```python
from build123d import *

# Parameters (mm, degrees)
SKETCH1_W           = 55.88
SKETCH1_H           = 9.981767046
SKETCH1_R           = 2.0193
BOSS_EXTRUDE1_DEPTH = 2.54
SKETCH2_W           = 55.88
SKETCH2_H           = 1.152145831
BOSS_EXTRUDE2_DEPTH = 17.78
SKETCH3_W           = 1.2265406
SKETCH3_H           = 17.78
SKETCH3_W_2         = 1.1438128
BOSS_EXTRUDE4_DEPTH = 6.35
SKETCH4_R           = 1.524
CUT_EXTRUDE1_DEPTH  = 105.035332272
CUT_EXTRUDE3_DEPTH  = 105.035332272
BOSS_EXTRUDE5_DEPTH = 2.54
BOSS_EXTRUDE6_DEPTH = 2.54
FILLET1_R           = 2.3368
FILLET2_R           = 2.3368
FILLET3_R           = 2.3368
FILLET4_R           = 2.3368
BOSS_EXTRUDE7_START = 2.54
SKETCH8_R           = 1.524
BOSS_EXTRUDE7_DEPTH = 2.54


with BuildPart() as part:
    # Sketch1 → Boss-Extrude1 (new body)
    with BuildSketch(Plane.XY):
        with Locations((-73.708835459, 211.206122276)):
            Rectangle(SKETCH1_W, SKETCH1_H)
        with Locations((-96.565388679, 211.879005799)):
            Circle(SKETCH1_R, mode=Mode.SUBTRACT)
        with Locations((-50.848835459, 211.879005799)):
            Circle(SKETCH1_R, mode=Mode.SUBTRACT)
    extrude(amount=BOSS_EXTRUDE1_DEPTH)

    # Sketch2 → Boss-Extrude2 (add)
    with BuildSketch(Plane.XY.offset(2.54)):
        with Locations((-73.708835459, 206.791311669)):
            Rectangle(SKETCH2_W, SKETCH2_H)
    extrude(amount=BOSS_EXTRUDE2_DEPTH)

    # Sketch3 → Boss-Extrude4 (add)
    with BuildSketch(Plane(origin=(0, 207.367384584, 0), x_dir=(1, 0, 0), z_dir=(0, 1, 0))):
        with Locations((-101.035565159, -11.43)):
            Rectangle(SKETCH3_W, SKETCH3_H)
        with Locations((-46.340741859, -11.43)):
            Rectangle(SKETCH3_W_2, SKETCH3_H)
    extrude(amount=BOSS_EXTRUDE4_DEPTH)

    # Sketch4 → Cut-Extrude1 (cut, through all)
    with BuildSketch(Plane(origin=(0, 207.367384584, 0), x_dir=(1, 0, 0), z_dir=(0, 1, 0))):
        with Locations(Location((-97.120294859, -13.7541, 0), (0, 0, 270))):
            Circle(SKETCH4_R)
        with Locations(Location((-50.214648259, -13.7541, 0), (0, 0, 270))):
            Circle(SKETCH4_R)
    extrude(amount=-CUT_EXTRUDE1_DEPTH, mode=Mode.SUBTRACT)

    # Sketch5 → Cut-Extrude3 (cut, through all)
    with BuildSketch(Plane(origin=(0, 207.367384584, 0), x_dir=(1, 0, 0), z_dir=(0, 1, 0))):
        Polygon((-53.474471559, -7.1501), (-93.860471559, -7.1501), (-95.795272253, -18.1229), (-95.795272253, -20.32), (-92.955896087, -20.32), (-62.921890572, -20.32), (-51.611648259, -20.32), (-51.611648259, -18.237455367), align=None)
    extrude(amount=-CUT_EXTRUDE3_DEPTH, mode=Mode.SUBTRACT)

    # Sketch6 → Boss-Extrude5 (add)
    with BuildSketch(Plane.ZY.offset(101.648835459)):
        Polygon((2.54, 216.197005799), (0, 216.197005799), (0, 206.215238753), (20.32, 206.215238753), (20.32, 213.717384584), (2.54, 213.717384584), align=None)
    extrude(amount=BOSS_EXTRUDE5_DEPTH)

    # Sketch7 → Boss-Extrude6 (add)
    with BuildSketch(Plane(origin=(-45.768835459, 0, 0), x_dir=(0, 0, -1), z_dir=(1, 0, 0))):
        Polygon((0, 216.197005799), (-2.54, 216.197005799), (-2.54, 213.717384584), (-20.32, 213.717384584), (-20.32, 206.215238753), (0, 206.215238753), align=None)
    extrude(amount=BOSS_EXTRUDE6_DEPTH)

    # Fillet1
    fillet1_edges = [part.edges().sort_by_distance(p)[0] for p in [
        (-93.860471559, 206.791311669, 7.1501),
    ]]
    fillet(fillet1_edges, radius=FILLET1_R)

    # Fillet2
    fillet2_edges = [part.edges().sort_by_distance(p)[0] for p in [
        (-53.474471559, 206.791311669, 7.1501),
    ]]
    fillet(fillet2_edges, radius=FILLET2_R)

    # Fillet3
    fillet3_edges = [part.edges().sort_by_distance(p)[0] for p in [
        (-95.795272253, 206.791311669, 18.1229),
    ]]
    fillet(fillet3_edges, radius=FILLET3_R)

    # Fillet4
    fillet4_edges = [part.edges().sort_by_distance(p)[0] for p in [
        (-51.611648259, 206.791311669, 18.237455367),
    ]]
    fillet(fillet4_edges, radius=FILLET4_R)

    # Sketch8 → Boss-Extrude7 (add)
    with BuildSketch(Plane.XZ.offset(-206.215238753).offset(BOSS_EXTRUDE7_START)):
        with BuildLine():
            Line((-55.451410668, 7.1501), (-91.899663541, 7.1501))
            ThreePointArc((-91.899663541, 7.1501), (-93.401729627, 7.696807345), (-94.200962298, 9.081118938))
            Line((-94.200962298, 9.081118938), (-95.75977101, 17.921562447))
            ThreePointArc((-95.75977101, 17.921562447), (-95.786380023, 18.123677969), (-95.795272253, 18.327343509))
            Line((-95.795272253, 18.327343509), (-95.795272253, 20.32))
            Line((-95.795272253, 20.32), (-104.188835459, 20.32))
            Line((-104.188835459, 20.32), (-104.188835459, 0))
            Line((-104.188835459, 0), (-43.228835459, 0))
            Line((-43.228835459, 0), (-43.228835459, 20.32))
            Line((-43.228835459, 20.32), (-51.611648259, 20.32))
            Line((-51.611648259, 20.32), (-51.611648259, 18.432395976))
            ThreePointArc((-51.611648259, 18.432395976), (-51.619737234, 18.238130166), (-51.64394816, 18.045209281))
            Line((-51.64394816, 18.045209281), (-53.14691057, 9.099713305))
            ThreePointArc((-53.14691057, 9.099713305), (-53.942129983, 7.702885971), (-55.451410668, 7.1501))
        make_face()
        with Locations(Location((-50.214648259, 13.7541, 0), (0, 0, 90))):
            Circle(SKETCH8_R, mode=Mode.SUBTRACT)
        with Locations(Location((-97.120294859, 13.7541, 0), (0, 0, 90))):
            Circle(SKETCH8_R, mode=Mode.SUBTRACT)
    extrude(amount=-BOSS_EXTRUDE7_DEPTH)


solid = part.part
```
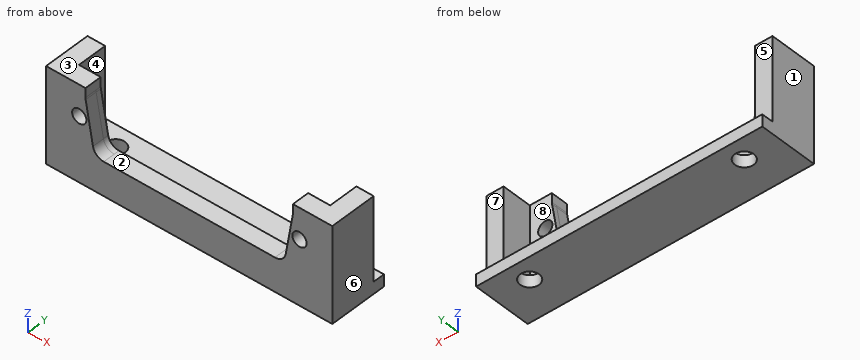
Part model, mm, in its own coordinate system. Face numbers are marked on the shaded views. A direction names the side the tool comes from. Coordinates: 2 decimals unless noted, no trailing zeros. Loops run counter-clockwise (first coordinate to the right, second up) from the corner with the lowest first, then second, coordinate; pieces in that order, holes last. Notation, with made-up numbers: (20, -32.5) - (76, -32.5) arc R29 cw to (76, 3.5) - close; hole circle Ø3 at (6.5, 65). An arc over 180 degrees is marked (long way). Write item = value, one per line. Start each with the question number.
Item 1: Cut at C-C, the plane x = -64.5. Give the cut face in (y, z).
Item 2: Mould opens along X. For the marked faces 6, 7 and 8 say: released by +X, released by -X, zero draft, split by the parting line, or undercut.
Item 3: Cut at B-B, the plane y = 208. Give the cut face in (x, z), and give its area (3 significant figures).
Item 4: Wall check: L1, parallel to X at y = 209.25, z = 7; L2, parallel to Z at x = -63, y = 212; L3, parallel to Y at x = -49, z = 15.5. Give the ranges that are in metal, low to high. Write a range as from..to.
Item 5: Flat gauge pins, fed straight in: pin 1 Ø4 at (x, y) = (-81, 214.5) entering from +Z; pin 2 Ø5.5 at (x, z) = (-76, 7) entering from +Y; pin 3 Ø3 at (x, z) = (-45, 12.5) entering from +Y. Where does each tip first touch, or does it go through?
Item 6: 3-axis set-ups, long thin cutter, end or side, ignore diameter. For the marked faces 1, 2, 3, 4 and 5: which of +Z, -Z, +X, -X, +Y, -Y reach the whole face in a straight line?
Item 7: Cut at A-A, the plane z = 13. Give the cut face in (x, y), and give its area (3 significant figures).
Item 8: Cut at D-D, the plane z = 16. Give the cut face in (x, y), and give its area (3 significant figures).
The answers:
q1.outline = (203.68, 0) - (216.2, 0) - (216.2, 2.54) - (207.37, 2.54) - (207.37, 7.15) - (203.68, 7.15) - close
q2.face_6 = released by +X
q2.face_7 = zero draft
q2.face_8 = undercut
q3.outline = (-104.19, 0) - (-43.23, 0) - (-43.23, 20.32) - (-46.91, 20.32) - (-46.91, 2.54) - (-100.42, 2.54) - (-100.42, 20.32) - (-104.19, 20.32) - close
q3.area = 287 mm2
q4.L1 = -104.19..-100.42, -46.91..-43.23
q4.L2 = 0..2.54
q4.L3 = 203.68..207.37
q5.pin_1 = 2.54
q5.pin_2 = 207.37
q5.pin_3 = 213.72
q6.face_1 = +Z, -Z, -X, +Y, -Y
q6.face_2 = +Z, +Y, -Y
q6.face_3 = +Z, +X, -X, +Y, -Y
q6.face_4 = +Z, +Y
q6.face_5 = +Z, +X, -X, +Y
q7.outline = (-104.19, 203.68) - (-98.44, 203.68) - (-98.44, 207.37) - (-100.42, 207.37) - (-100.42, 213.72) - (-104.19, 213.72) - close; (-95.8, 203.68) - (-94.89, 203.68) - (-94.89, 207.37) - (-95.8, 207.37) - close; (-52.49, 203.68) - (-51.54, 203.68) - (-51.54, 207.37) - (-52.49, 207.37) - close; (-48.89, 203.68) - (-43.23, 203.68) - (-43.23, 213.72) - (-46.91, 213.72) - (-46.91, 207.37) - (-48.89, 207.37) - close
q7.area = 96.3 mm2
q8.outline = (-104.19, 203.68) - (-95.42, 203.68) - (-95.42, 207.37) - (-100.42, 207.37) - (-100.42, 213.72) - (-104.19, 213.72) - close; (-51.99, 203.68) - (-43.23, 203.68) - (-43.23, 213.72) - (-46.91, 213.72) - (-46.91, 207.37) - (-51.99, 207.37) - close
q8.area = 112 mm2
